Here's how the part is built. I have some questions about the finished solid (model axes, mm). A direction names the side the tool comes from. Coordinates: 2 decimals unless noted, no trailing zeros. Write each loop counter-clockwise with the first axis right and the second up, starting at its lowest first coordinate (ties: lowest second). Pieces come first, ordered by that corner, then holes.
```python
from build123d import *

# Parameters (mm, degrees)
SKETCH1_W           = 12
SKETCH1_H           = 7
BOSS_EXTRUDE1_DEPTH = 2
SKETCH3_W           = 1.5
SKETCH3_H           = 1
CUT_EXTRUDE1_DEPTH  = 4
LPATTERN1_COUNT     = 6
LPATTERN1_PITCH     = 1.9


with BuildPart() as part:
    # Sketch1 → Boss-Extrude1 (new body)
    with BuildSketch(Plane.XY):
        with Locations((6, 3.5)):
            Rectangle(SKETCH1_W, SKETCH1_H)
    extrude(amount=BOSS_EXTRUDE1_DEPTH)

    # Sketch3 → Cut-Extrude1 (cut)
    with BuildSketch(Plane(origin=(0, 7, 0), x_dir=(1, 0, 0), z_dir=(0, 1, 0))):
        with Locations((1.263938608, -1)):
            Rectangle(SKETCH3_W, SKETCH3_H)
    cut_extrude1 = extrude(amount=-CUT_EXTRUDE1_DEPTH, mode=Mode.SUBTRACT)

    # LPattern1: Cut-Extrude1 ×6
    with Locations(*[(i * LPATTERN1_PITCH, 0, 0) for i in range(1, LPATTERN1_COUNT)]):
        add(cut_extrude1, mode=Mode.SUBTRACT)


solid = part.part
```
1) Imagine slicing it at B-B on x = 9. Please give me the cut outline in (y, z).
Values follow:
outline: (0, 0) - (7, 0) - (7, 0.5) - (3, 0.5) - (3, 1.5) - (7, 1.5) - (7, 2) - (0, 2) - close
2) We'd pull the mould along Z, two halves only. Please class faces 1 (the face through (2.014, 5, 1)), 2 (the face through (6, 7, 1)): pulls with the +Z half, pulls with the -Z half, needs draft (parallel to the pull), parting line crosses it, or undercut.
Values follow:
face 1: undercut
face 2: needs draft
3) Imagine slicing it at A-A on y = 3.5. Please give me the cut outline in (x, z), then the cut area to 3 significant figures.
Values follow:
outline: (0, 0) - (12, 0) - (12, 2) - (0, 2) - close; hole (0.51, 0.5) - (2.01, 0.5) - (2.01, 1.5) - (0.51, 1.5) - close; hole (2.41, 0.5) - (3.91, 0.5) - (3.91, 1.5) - (2.41, 1.5) - close; hole (4.31, 0.5) - (5.81, 0.5) - (5.81, 1.5) - (4.31, 1.5) - close; hole (6.21, 0.5) - (7.71, 0.5) - (7.71, 1.5) - (6.21, 1.5) - close; hole (8.11, 0.5) - (9.61, 0.5) - (9.61, 1.5) - (8.11, 1.5) - close; hole (10.01, 0.5) - (11.51, 0.5) - (11.51, 1.5) - (10.01, 1.5) - close
area: 15.0 mm2
4) On a 3-axis mill with a long thin cutter (end or side, diameter ignored), from which of +Z, -Z, +X, -X, +Y, -Y can I reach the whole of each face in a straight line? I mean faces 3 (the face through (12, 3, 1)), 4 (the face through (5, 5, 0.5)). Say none if no direction works.
Values follow:
face 3: +Z, -Z, +X, +Y, -Y
face 4: +Y
5) I need wall thicknesses on probe 1 along Z at (x, y) = (5.75, 5.5); probe 2 along Y at (x, z) = (4.75, 0.8). Which ranges of each line are inside material? Lowest first, please.
Values follow:
probe 1: z = 0 to 0.5, 1.5 to 2
probe 2: y = 0 to 3
6) Imagine slicing it at C-C on z = 1.35. Please give me the cut outline in (x, y).
Values follow:
outline: (0, 0) - (12, 0) - (12, 7) - (11.51, 7) - (11.51, 3) - (10.01, 3) - (10.01, 7) - (9.61, 7) - (9.61, 3) - (8.11, 3) - (8.11, 7) - (7.71, 7) - (7.71, 3) - (6.21, 3) - (6.21, 7) - (5.81, 7) - (5.81, 3) - (4.31, 3) - (4.31, 7) - (3.91, 7) - (3.91, 3) - (2.41, 3) - (2.41, 7) - (2.01, 7) - (2.01, 3) - (0.51, 3) - (0.51, 7) - (0, 7) - close
